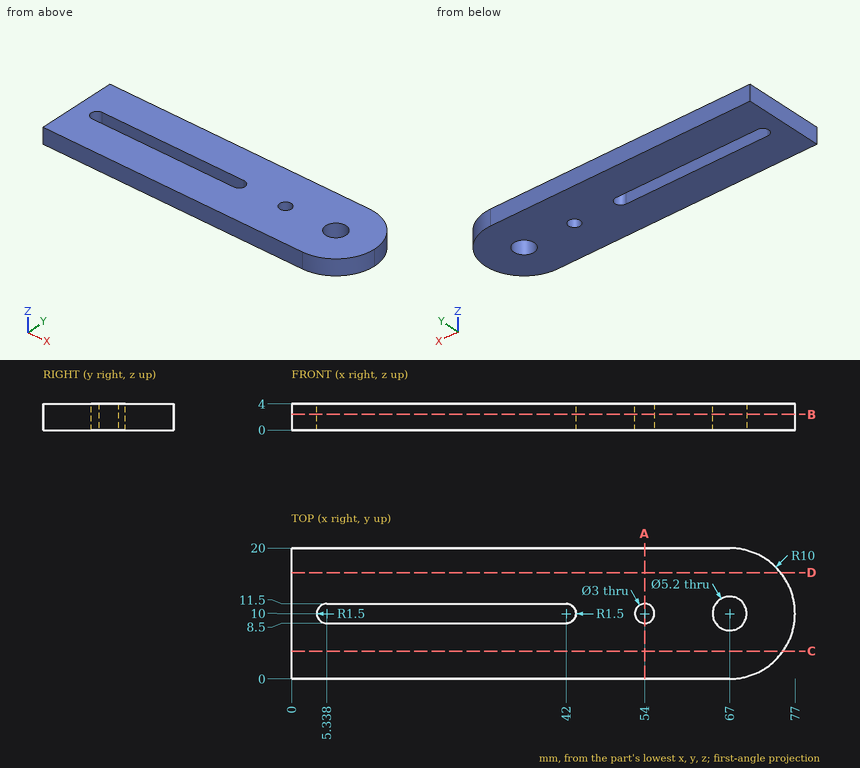
For this review, use the dimensioned drawing (mm, ordinates from the lowest corner) and the shaded views. Round coordinates to 2 decimals unless told otherwise and drop trailing zeros. Loops run counter-clockwise (first coordinate to the right, second up) from the corner with the lowest first, then second, coordinate; pieces in that order, holes last. Notation, with made-up numbers: (50.5, 51.5) -> (55.5, 51.5) arc R37 ccw to (55.5, 87.5) -> close; hole circle Ø8 at (49, 42). An arc over 180 degrees is marked (long way). Write item = value, one per line. Start each with the question number.
Item 1: Take a section at C-C on y = 4.25. Give the boundary of the cut face in (x, z), plus the area to 3 significant figures.
Item 2: Take a section at D-D on y = 16.25. Give the boundary of the cut face in (x, z).
Item 3: Insertion check: pin 1 (1.2 mm diameter, centred on x = 17.5, z = 2.5, fed in from -Y); pin 2 (1.5 mm diameter, centred on y = 7.5, z = 2.5, fed in from +X). Each pin has a flat end and moves straight along its axis. Give the tip position at first contact, or say it passes through.
Item 4: Take a section at A-A on x = 54. Give the boundary of the cut face in (y, z), plus the area to 3 significant figures.
Item 5: Take a section at B-B on z = 2.4. Give the boundary of the cut face in (x, y), plus the area to 3 significant figures.
Item 6: To check wall thickness, follow L1, parallel to Y at x = 54, z = 2.9; L2, parallel to Y at x = 67, z = 0.9; L3, parallel to X at y = 9.5, z = 2.3 (1 decimal). State the ranges of each line that lie inside material, in increasing order.
Result:
q1.outline = (0, 0) -> (75.18, 0) -> (75.18, 4) -> (0, 4) -> close
q1.area = 301 mm²
q2.outline = (0, 0) -> (74.81, 0) -> (74.81, 4) -> (0, 4) -> close
q3.pin_1 = 0
q3.pin_2 = 76.85
q4.outline = (0, 0) -> (8.5, 0) -> (8.5, 4) -> (0, 4) -> close; (11.5, 0) -> (20, 0) -> (20, 4) -> (11.5, 4) -> close
q4.area = 68.0 mm²
q5.outline = (0, 0) -> (67, 0) arc R10 ccw to (67, 20) -> (0, 20) -> close; hole (5.34, 8.5) -> (42, 8.5) arc R1.5 ccw to (42, 11.5) -> (5.34, 11.5) arc R1.5 ccw to start; hole circle Ø3 at (54, 10); hole circle Ø5.2 at (67, 10)
q5.area = 1,350 mm²
q6.L1 = 0 to 8.5, 11.5 to 20
q6.L2 = 0 to 7.4, 12.6 to 20
q6.L3 = 0 to 3.9, 43.4 to 52.6, 55.4 to 64.4, 69.6 to 77
